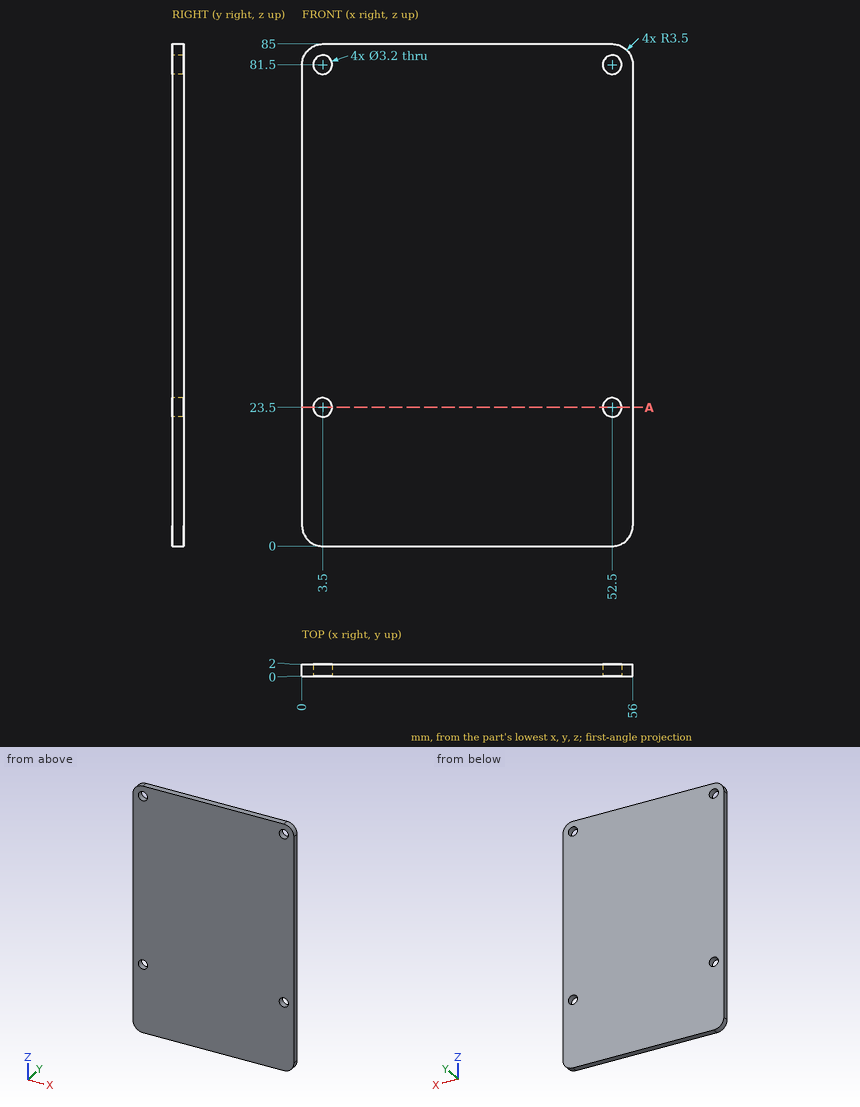
Answer from the drawing. Dimensions are ordinates in mm from the lowest x, y and z of the part. Give positions to 0.01 mm unless a question says otherwise; leave off trailing zeros. Loops run counter-clockwise (first coordinate to the right, second up) from the corner with the lowest first, then second, coordinate; pieces in that order, holes last. Notation, with made-up numbers: (32, 32.5) - (47, 32.5) arc R22 ccw to (47, 43.5) - close; hole circle Ø7 at (-31.5, 60.25). An arc over 180 degrees is marked (long way). Answer as a JSON object with one key per item and string values.
1. A flat-ended cylindrical pin translates along its axis: pin 1 Ø3 at (x, z) = (52.5, 23.5) entering from -Y. Find the tip coordinate at first contact, or state that the pin passes through.
Determined:
{"pin 1": "through"}
2. A cutting plane is placed at A-A (z = 23.5). Write down the section's boundary in (x, y), then the cut area to 3 significant figures.
Determined:
{"outline": "(0, 0) - (1.9, 0) - (1.9, 2) - (0, 2) - close; (5.1, 0) - (50.9, 0) - (50.9, 2) - (5.1, 2) - close; (54.1, 0) - (56, 0) - (56, 2) - (54.1, 2) - close", "area": "99.2 mm²"}
3. Find the intervals of material crossed by L1, parallel to X at y = 1, z = 23.5; L2, parallel to Z at x = 3.5, y = 1.4, in increasing order. Write a range as [from, to].
Determined:
{"L1": "[0, 1.9], [5.1, 50.9], [54.1, 56]", "L2": "[0, 21.9], [25.1, 79.9], [83.1, 85]"}
